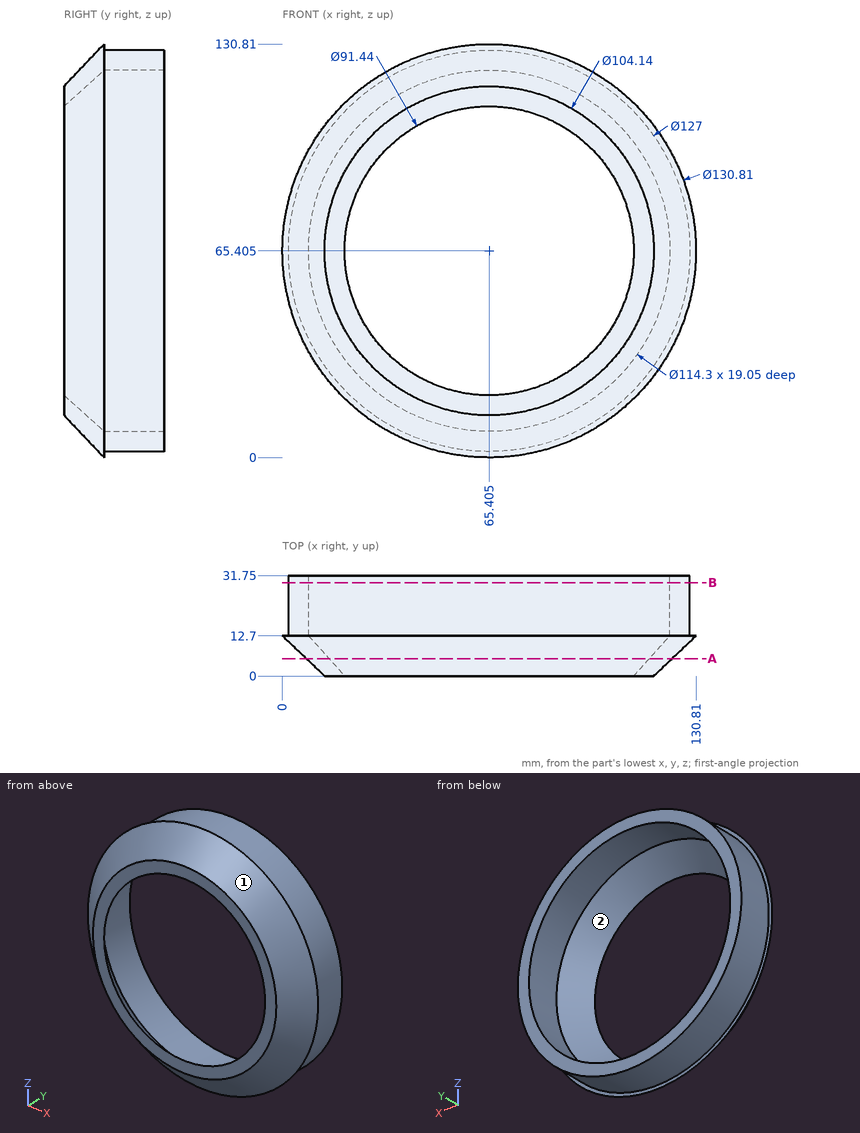
Geometry: see drawing. Coordinates: mm, zero at the bounding-box minimum. Give positions to 0.01 mm unless a question says otherwise; leave off trailing zeros. Loops run counter-clockwise (first coordinate to the right, second up) from the corner with the lowest first, then second, coordinate; pieces in that order, holes last. Notation, with made-up numbers: M -17.75,-13.75 L 7.25,-13.75 A9 ccw 7.25,-4.75 Z; hole C 33,-36.5 d10. An arc over 180 degrees is marked long. Use one line per item in the form item = value.
1. Section query B-B, the plane y = 29.5. Return the cut outline in (x, z) (3 decimals), and give its area (3 significant figures).
Numbers:
outline = C 65.405,65.405 d127; hole C 65.405,65.405 d114.3
area = 2,410 mm²
2. Line query: L1, parallel to X at y = 16.5, z = 49.5; L2, parallel to Z at x = 89.5, y = 22; L3, parallel to X at y = 15, z = 104. Output: solid intervals per line, ascending.
Numbers:
L1 = 3.93 to 10.51, 120.3 to 126.88
L2 = 6.65 to 13.58, 117.23 to 124.16
L3 = 14.98 to 23.26, 107.55 to 115.83
3. Pull-direction query (X, two-part tool) for the marked faces 1 and 2; classes: released by +X, released by -X, zero draft, split by the parting line, or undercut.
Numbers:
face_1 = split by the parting line
face_2 = undercut
4. First-contact query: pin 1 (6 mm diameter, centred on y = 21.5, z = 67.5, fed in from +X) (3 decimals); pin 2 (2 mm diameter, centred on x = 15, y = 27.5, fed in from +Z); pin 3 (12 mm diameter, centred on x = 102, y = 10.5, fed in from -Z). Flat tips, straight axial feed; report the tip coordinate or a pass-through.
Numbers:
pin_1 = 128.905
pin_2 = 105.3
pin_3 = 7.82
5. Section query A-A, the plane y = 5.5. Return the cut outline in (x, z) (3 decimals), and give its area (3 significant figures).
Numbers:
outline = C 65.405,65.405 d115.69; hole C 65.405,65.405 d101.34
area = 2,450 mm²
